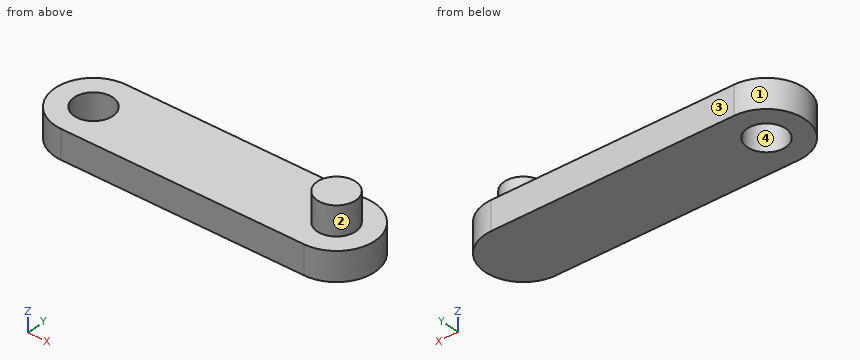
```python
from build123d import *

# Parameters (mm, degrees)
SKETCH2_R           = 20
BOSS_EXTRUDE1_DEPTH = 30
SKETCH7_R           = 20
BOSS_EXTRUDE2_DEPTH = 30


with BuildPart() as part:
    # Sketch2 → Boss-Extrude1 (new body)
    with BuildSketch(Plane.XY):
        with BuildLine():
            Line((0, 0), (250, 0))
            ThreePointArc((250, 0), (290, -40), (250, -80))
            Line((250, -80), (0, -80))
            ThreePointArc((0, -80), (-40, -40), (0, 0))
        make_face()
        with Locations((0, -40)):
            Circle(SKETCH2_R, mode=Mode.SUBTRACT)
    extrude(amount=BOSS_EXTRUDE1_DEPTH)

    # Sketch7 → Boss-Extrude2 (add)
    with BuildSketch(Plane.XY.offset(30)):
        with Locations((250, -40)):
            Circle(SKETCH7_R)
    extrude(amount=BOSS_EXTRUDE2_DEPTH)


solid = part.part
```
Here's how the part is built. I have some questions about the finished solid (model axes, mm). Face numbers are marked on the shaded views. Coordinates: 2 decimals unless noted, no trailing zeros. Loops run counter-clockwise (first coordinate to the right, second up) from the corner with the lowest first, then second, coordinate; pieces in that order, holes last. Notation, with made-up numbers: (20.5, 5.25) - (71.5, 5.25) arc R8 ccw to (71.5, 13.25) - close; hole circle Ø2 at (-21.5, -34). An arc over 180 degrees is marked (long way). Return JSON: item names as keys, results as strings. Group by question number.
Item 1: If we section it at B-B on z = 18: Write out the boundary of the cut face in (x, y).
Item 2: We'd pull the mould along X, two halves only. Please class the marked faces 1, 2, 3 and 4: +X half, -X half, draft (parallel to the pull), parting line (faces both ways), or undercut.
Item 3: If we section it at A-A on y = -40: Write out the boundary of the cut face in (x, z).
Item 4: I need wall thicknesses on line 1 (Y direction, x = 0, z = 18.25); line 2 (Z direction, x = 275.5, y = -56); line 3 (X direction, y = -36, z = 4). Which ranges of each line are inside material? Lowest first, please. Write a range as from..to.
Item 5: If we section it at D-D on x = 90: Write out the boundary of the cut face in (y, z).
Item 6: Will these pins go through, and if not, where does the flat tip stop? P1, Ø3, axis at x = 251.5, z = 6, coming from the -Y side; P2, Ø12, axis at x = 65, y = -66, coming from the +Z side; P3, Ø3, axis at y = -64, z = 23.5, coming from the +X side; P4, Ø1, axis at y = -53, z = 32.5, coming from the +X side.
Item 7: If we section it at C-C on y = -24: Write out the boundary of the cut face in (x, z).
Calculated:
{
 "1": {"outline": "(0, -80) - (250, -80) arc R40 ccw to (250, 0) - (0, 0) arc R40 ccw to start; hole circle Ø40 at (0, -40)"},
 "2": {"face 1": "-X half", "face 2": "parting line", "face 3": "draft", "face 4": "undercut"},
 "3": {"outline": "(-40, 0) - (-20, 0) - (-20, 30) - (-40, 30) - close; (20, 0) - (290, 0) - (290, 30) - (270, 30) - (270, 60) - (230, 60) - (230, 30) - (20, 30) - close"},
 "4": {"line 1": "y = -80..-60, -20..0", "line 2": "z = 0..30", "line 3": "x = -39.8..-19.6, 19.6..289.8"},
 "5": {"outline": "(-80, 0) - (0, 0) - (0, 30) - (-80, 30) - close"},
 "6": {"P1": "stops at y = -80", "P2": "stops at z = 30", "P3": "stops at x = 283.07", "P4": "stops at x = 265.61"},
 "7": {"outline": "(-36.66, 0) - (-12, 0) - (-12, 30) - (-36.66, 30) - close; (12, 0) - (286.66, 0) - (286.66, 30) - (262, 30) - (262, 60) - (238, 60) - (238, 30) - (12, 30) - close"}
}
